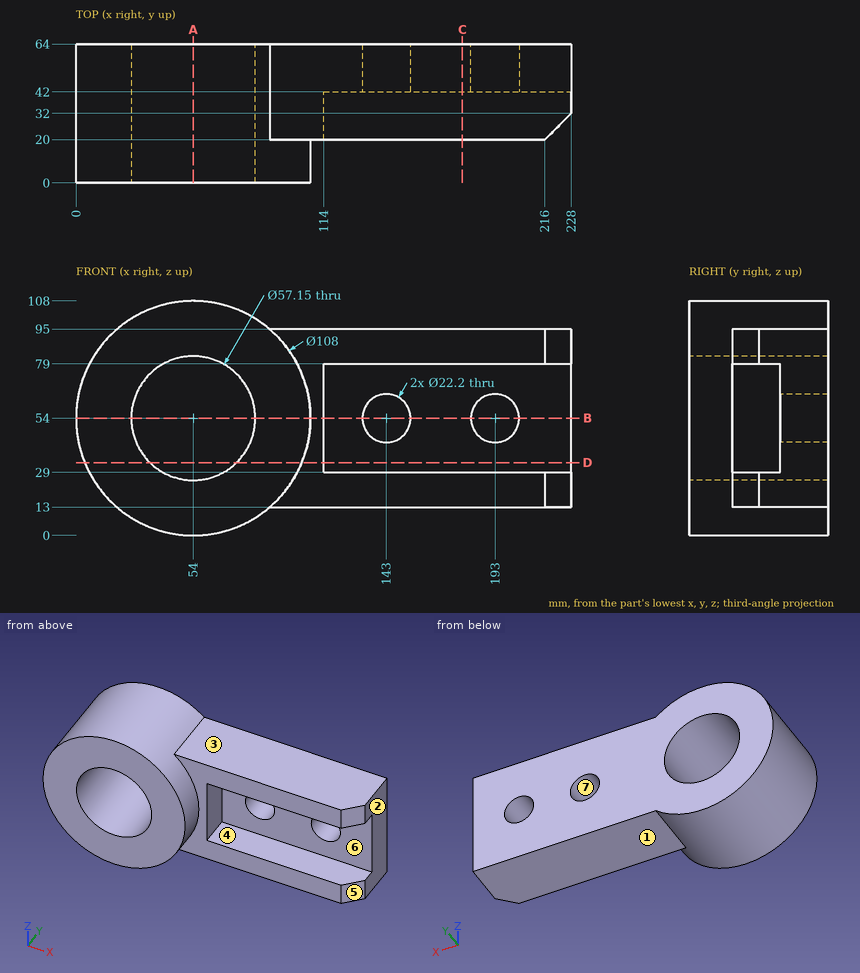
Geometry: see drawing. Coordinates: mm, zero at the bounding-box minimum. A direction names the side the tool comes from. Give positions to 0.01 mm unless a question says otherwise; leave off trailing zeros. Order: outer loops, then holes, each group sorted by start corner. A loop starts at its lowest first (then second) coordinate and runs counter-clockwise, first axis right, second up. Notation, with made-up numbers: (5.5, -24.5) - (64.5, -24.5) arc R28 cw to (64.5, 9.5) - close; hole circle Ø1 at (80, -4.5). An arc over 180 degrees is marked (long way). Use a Markdown table: item, result.
(1) Draft query along X for the marked faces 5, 6 and 7. Return one class per face: released by +X, released by -X, zero draft, split by the parting line, or undercut.
Computed values:
| item | result |
|---|---|
| face 5 | released by +X |
| face 6 | zero draft |
| face 7 | undercut |
(2) Line query: line 1 (Z direction, x = 54.5, y = 34); line 2 (X direction, y = 60.5, z = 50); line 3 (Z direction, x = 143, y = 51). Output: solid intervals per line, ascending. Write a range as from..to.
Computed values:
| item | result |
|---|---|
| line 1 | z = 0..25.43, 82.57..108 |
| line 2 | x = 0.15..25.71, 82.29..132.65, 153.35..182.65, 203.35..228 |
| line 3 | z = 13..42.9, 65.1..95 |
(3) Section query B-B (z = 54). Output: boundary loops of the cut face in (x, y) (3 decimals), then the cut area to 3 significant figures.
Computed values:
| item | result |
|---|---|
| outline | (0, 0) - (25.425, 0) - (25.425, 64) - (0, 64) - close; (82.575, 0) - (108, 0) - (108, 20) - (114, 20) - (114, 42) - (131.9, 42) - (131.9, 64) - (82.575, 64) - close; (154.1, 42) - (181.9, 42) - (181.9, 64) - (154.1, 64) - close; (204.1, 42) - (228, 42) - (228, 64) - (204.1, 64) - close |
| area | 5,050 mm2 |
(4) Access query for the marked faces 1, 2, 3 and 4. Directions: +Z, -Z, +X, -X, +Y, -Y. A direction counts if a zero-diameter tool reaches every point of the face in a straight line with its end or side. Return the directions, or none.
Computed values:
| item | result |
|---|---|
| face 1 | -Z, +X, +Y, -Y |
| face 2 | +Z, -Z, +X, +Y, -Y |
| face 3 | +Z, +X, +Y, -Y |
| face 4 | +X, -Y |
(5) Section query C-C (x = 178). Output: boundary loops of the cut face in (y, z), then the cut area to 3 significant figures.
Computed values:
| item | result |
|---|---|
| outline | (20, 13) - (64, 13) - (64, 95) - (20, 95) - (20, 79) - (42, 79) - (42, 29) - (20, 29) - close |
| area | 2,510 mm2 |
(6) Section query D-D (z = 33.5). Output: boundary loops of the cut face in (x, y).
Computed values:
| item | result |
|---|---|
| outline | (4.04, 0) - (34.09, 0) - (34.09, 64) - (4.04, 64) - close; (73.91, 0) - (103.96, 0) - (103.96, 20) - (114, 20) - (114, 42) - (228, 42) - (228, 64) - (73.91, 64) - close |
(7) Pin query (flat end, axial travel): pin 1 (24.5 mm diameter, centred on x = 158, z = 60.5, fed in from -Y); pin 2 (18 mm diameter, centred on x = 143, z = 54, fed in from +Y); pin 3 (11 mm diameter, centred on y = 34, z = 65, fed in from +X); pin 4 (17.5 mm diameter, centred on x = 168, y = 32, fed in from +Z). Return the tip coordinate at first contact, or that it passes through.
Computed values:
| item | result |
|---|---|
| pin 1 | stops at y = 42 |
| pin 2 | passes through |
| pin 3 | stops at x = 114 |
| pin 4 | stops at z = 95 |
(8) Section query A-A (x = 54). Output: boundary loops of the cut face in (y, z) (3 decimals).
Computed values:
| item | result |
|---|---|
| outline | (0, 0) - (64, 0) - (64, 25.425) - (0, 25.425) - close; (0, 82.575) - (64, 82.575) - (64, 108) - (0, 108) - close |
